Here's the drawing with two shaded views (mm, measured from the low corner). I have some questions. A direction names the side the tool comes from. Give positions to 0.01 mm unless a question says otherwise; leave off trailing zeros. Write each loop counter-clockwise with the first axis right and the second up, starting at its lowest first coordinate (ties: lowest second). Pieces come first, ordered by that corner, then holes. Notation, with made-up numbers: (83.5, 51) - (90.5, 51) arc R15 ccw to (90.5, 63) - close; hole circle Ø4 at (79.25, -32). An arc over 180 degrees is marked (long way). Use one line per item in the form item = value.
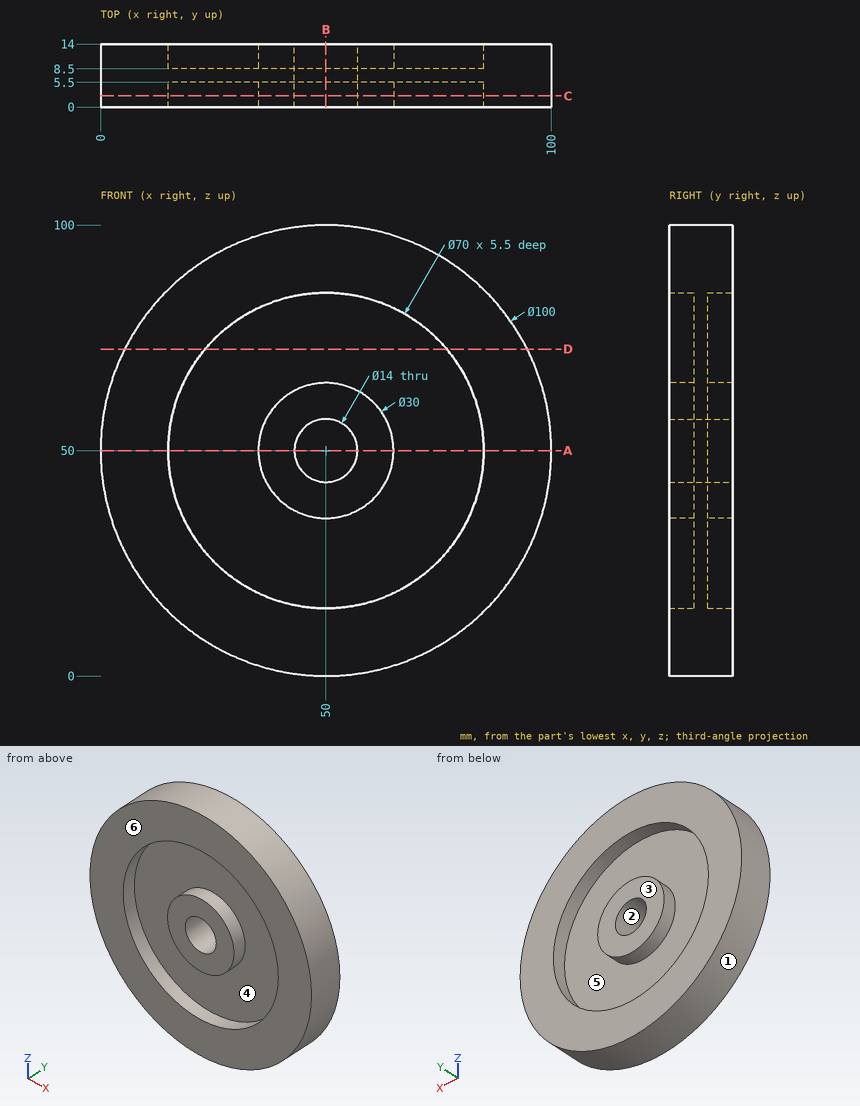
1. Imagine slicing it at B-B, the plane x = 50. List the corners of the cut face in (y, z) for me.
Response values:
outline = (0, 0) - (14, 0) - (14, 15) - (8.5, 15) - (8.5, 35) - (14, 35) - (14, 43) - (0, 43) - (0, 35) - (5.5, 35) - (5.5, 15) - (0, 15) - close; (0, 57) - (14, 57) - (14, 65) - (8.5, 65) - (8.5, 85) - (14, 85) - (14, 100) - (0, 100) - (0, 85) - (5.5, 85) - (5.5, 65) - (0, 65) - close
2. If I drill on line 1 (Z direction, x = 50, y = 10.2); line 2 (Z direction, x = 50, y = 7); line 3 (X direction, y = 3.25, z = 47), over which ranges is the centre line in solid material (lowest first)? Write a range as from..to.
Response values:
line_1 = 0..15, 35..43, 57..65, 85..100
line_2 = 0..43, 57..100
line_3 = 0.09..15.13, 35.3..43.68, 56.32..64.7, 84.87..99.91
3. For pin 1 (8.5 mm diameter, centred on x = 50, z = 50, fed in from -Y); pin 2 (8 mm diameter, centred on x = 71, y = 10.5, fed in from -Z); pin 3 (2 mm diameter, centred on x = 86.5, y = 7.5, fed in from -Z); pin 4 (1 mm diameter, centred on x = 26, y = 12, fed in from -Z), each with a flat end and sliding along its axis, tell me the tip position at first contact or that it passes through.
Response values:
pin_1 = through
pin_2 = 2.98
pin_3 = 14.79
pin_4 = 5.87
4. If we mould it in two halves opening along X, with no side actions, what happens to the marked faces 1, 2 and 3? For each: pulls with the +X half, pulls with the -X half, needs draft (parallel to the pull), parting line crosses it, or undercut.
Response values:
face_1 = parting line crosses it
face_2 = undercut
face_3 = needs draft
5. Imagine slicing it at C-C, the plane y = 2.5. List the corners of the cut face in (x, z) for me.
Response values:
outline = circle Ø100 at (50, 50); circle Ø30 at (50, 50); hole circle Ø70 at (50, 50); hole circle Ø14 at (50, 50)
6. Imagine slicing it at A-A, the plane z = 50. List the corners of the cut face in (x, y) for me.
Response values:
outline = (0, 0) - (15, 0) - (15, 5.5) - (35, 5.5) - (35, 0) - (43, 0) - (43, 14) - (35, 14) - (35, 8.5) - (15, 8.5) - (15, 14) - (0, 14) - close; (57, 0) - (65, 0) - (65, 5.5) - (85, 5.5) - (85, 0) - (100, 0) - (100, 14) - (85, 14) - (85, 8.5) - (65, 8.5) - (65, 14) - (57, 14) - close
7. Imagine slicing it at D-D, the plane z = 72.5. List the corners of the cut face in (x, y) for me.
Response values:
outline = (5.35, 0) - (23.19, 0) - (23.19, 5.5) - (76.81, 5.5) - (76.81, 0) - (94.65, 0) - (94.65, 14) - (76.81, 14) - (76.81, 8.5) - (23.19, 8.5) - (23.19, 14) - (5.35, 14) - close
8. Which directions (+Z, -Z, +X, -X, +Y, -Y) give clear straight access to the entire face, cutting with the end or side of a thin tool? Please do the marked faces 4, 5 and 6.
Response values:
face_4 = -Y
face_5 = +Y
face_6 = +Z, -Z, +X, -X, -Y
